The model under review builds one solid part; all positions refer to its coordinate system, in mm. A direction names the side the tool comes from. Round coordinates to 2 decimals unless told otherwise and drop trailing zeros. Order: outer loops, then holes, each group sorted by start corner. A loop starts at its lowest first (then second) coordinate and runs counter-clockwise, first axis right, second up.
Autodesk Inventor part; units mm, degrees
ref_plane "YZ Plane" through (0, 0, 0) normal (1, 0, 0) x (0, 1, 0)
ref_plane "XZ Plane" through (0, 0, 0) normal (0, 1, 0) x (-1, 0, 0)
ref_plane "XY Plane" through (0, 0, 0) normal (0, 0, 1) x (1, 0, 0)
sketch "Sketch1" plane through (0, 0, 0) normal (1, 0, 0) x (0, 1, 0)
  line L0 (0, 0) -> (3.9688, 0) construction
  line L1 (3.9688, 0) -> (3.9687, 19.05)
  line L2 (3.9687, 19.05) -> (0, 19.05) construction
  line L3 (0, 19.05) -> (0, 0) construction
  line L4 (3.9688, 0) -> (6.35, 0)
  line L5 (6.35, 0) -> (6.35, 19.05)
  line L6 (6.35, 19.05) -> (3.9687, 19.05)
  line L7 (3.9687, 19.05) -> (3.9688, 0)
  line L8 (6.35, 0) -> (8.7313, 0)
  line L9 (8.7313, 0) -> (8.7312, 6.35)
  line L10 (8.7312, 6.35) -> (6.35, 6.35)
  line L11 (6.35, 6.35) -> (6.35, 0)
  line L12 (6.35, 19.05) -> (8.7312, 19.05)
  line L13 (8.7312, 19.05) -> (8.7312, 15.875)
  line L14 (8.7312, 15.875) -> (6.35, 15.875)
  line L15 (6.35, 15.875) -> (6.35, 19.05)
  point P0 (6.35, 6.35)
  point P1 (6.35, 15.875)
  dimension "d0" = 3.9688
  dimension "d1" = 19.05
  dimension "d2" = 2.3813
  dimension "d3" = 2.3813
  dimension "d4" = 6.35
  dimension "d5" = 2.3813
  dimension "d8" = 9.525
revolve "Revolution1" add sketch "Sketch1" angle 360 about axis through (0, 0, 19.05) along (0, 0, -1)
chamfer "Chamfer1" distance 0.5 angle 45 3 edges at (0, -8.7313, 0) (0, -8.7312, 6.35) (0, -8.7312, 15.875)
equation "\"d5\" = d3"
properties part number "Spring Anchor" material "Nylon 6/6"
(1) Consider section C-C (z = 17.75). Write out the cut boundary in (x, y).
Data:
outline: circle Ø17.46 at (0, 0); hole circle Ø7.94 at (0, 0)
(2) To check wall thickness, follow probe 1 along X at (y, z) = (0, 7); probe 2 along Z at (x, y) = (-2, -6.5) (3 decimals); probe 3 along X at (y, z) = (-3, 4.25). State the ranges of each line that lie inside material, in increasing order.
Data:
probe 1: x = -6.35 to -3.97, 3.97 to 6.35
probe 2: z = 0 to 6.35, 15.875 to 19.05
probe 3: x = -8.2 to -2.6, 2.6 to 8.2
(3) Consider section A-A (x = 0). Write out the cut boundary in (y, z) (3 decimals).
Data:
outline: (-8.731, 0.5) - (-8.231, 0) - (-3.969, 0) - (-3.969, 19.05) - (-8.731, 19.05) - (-8.731, 16.375) - (-8.231, 15.875) - (-6.35, 15.875) - (-6.35, 6.35) - (-8.231, 6.35) - (-8.731, 5.85) - close; (3.969, 0) - (8.231, 0) - (8.731, 0.5) - (8.731, 5.85) - (8.231, 6.35) - (6.35, 6.35) - (6.35, 15.875) - (8.231, 15.875) - (8.731, 16.375) - (8.731, 19.05) - (3.969, 19.05) - close
(4) Draft analysis for pull direction X (two halves, no side actions). For faces 3 (the cylindrical face through (6.2, -1.38, 11.18)), 4 (the cylindrical face through (1.52, 3.666, 9.658)), 5 (the flat face through (2, 4, 0)), state which applies: pulls with the +X half, pulls with the -X half, needs draft (parallel to the pull), parting line crosses it, or undercut.
Data:
face 3: parting line crosses it
face 4: undercut
face 5: needs draft
(5) For faces 1 (the flat face through (-2, 4, 19.05)), 2 (the flat face through (-6.1, 2.4, 15.875)), list the 3-axis set-ups (+Z, -Z, +X, -X, +Y, -Y) from which the entire face can be reached by the end or side of a thin tool; tool diameter is ignored.
Data:
face 1: +Z, +X, -X, +Y, -Y
face 2: none
(6) Consider section D-D (z = 12.75). Write out the cut boundary in (x, y), and give its area (3 significant figures).
Data:
outline: circle Ø12.7 at (0, 0); hole circle Ø7.94 at (0, 0)
area: 77.2 mm2
(7) Insertion check: pin 1 (7 mm diameter, centred on x = 0, y = 0, fed in from -Z); pin 2 (10 mm diameter, centred on y = 6, z = 11, fed in from +X); pin 3 (8 mm diameter, centred on x = 4.5, z = 9, fed in from +Y); pin 4 (4 mm diameter, centred on x = 1, z = 14.5, fed in from -Y). Each pin has a flat end and moves straight along its axis. Give the tip position at first contact, or say it passes through.
Data:
pin 1: passes through
pin 2: stops at x = 7.1
pin 3: stops at y = 8.49
pin 4: stops at y = -8.73
